For this review, take the finished solid that the model builds, in its own axes (mm). Coordinates: 2 decimals unless noted, no trailing zeros. Write each loop counter-clockwise with the first axis right and the second up, starting at its lowest first coordinate (ties: lowest second). Pieces come first, ordered by that corner, then holes. Notation, with made-up numbers: M 51,-26 L 97,-26 A13 cw 97,-16 Z; hole C -4,15 d2. An arc over 180 degrees is marked long. One line per question, with ' | ' between items.
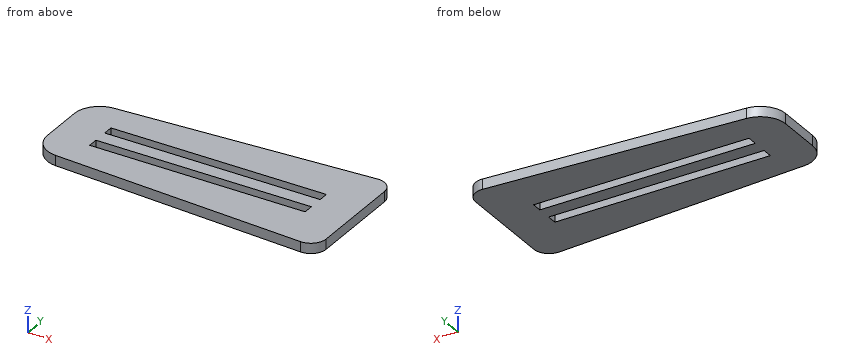
from build123d import *

# Parameters (mm, degrees)
F0_W     = 42.4481438452
F0_H     = 2
F1_DEPTH = 2
F2_R     = 3
F3_R     = 5


with BuildPart() as f1:
    # F0 (on Top) → F1 (new body)
    with BuildSketch(Plane.XY):
        Polygon((-65.7136544558, 44.0634722376), (-65.7136544558, 36.4734722376), (-65.7136544558, 35.0634722376), (-65.7136544558, 33.6534722376), (-65.7136544558, 26.0634722376), (-7.7136544558, 22.5634722376), (-7.7136544558, 47.5634722376), align=None)
        with Locations((-36.7136544558, 32.6534722376)):
            Rectangle(F0_W, F0_H, mode=Mode.SUBTRACT)
        with Locations((-36.7136544558, 37.4734722376)):
            Rectangle(F0_W, F0_H, mode=Mode.SUBTRACT)
    extrude(amount=F1_DEPTH)

    # F2
    f2_edges = [f1.edges().sort_by_distance(p)[0] for p in [
        (-7.713654, 47.563472, 1),
        (-7.713654, 22.563472, 1),
    ]]
    fillet(f2_edges, radius=F2_R)

    # F3
    f3_edges = [f1.edges().sort_by_distance(p)[0] for p in [
        (-65.713654, 26.063472, 1),
        (-65.713654, 44.063472, 1),
    ]]
    fillet(f3_edges, radius=F3_R)


solid = f1.part
1) We need section A-A on y = 37.5. State the section outline as (x, z) points, then the cut area to 3 significant figures.
Responses:
outline: M -65.71,0 L -57.94,0 L -57.94,2 L -65.71,2 Z; M -15.49,0 L -7.71,0 L -7.71,2 L -15.49,2 Z | area: 31.1 mm^2
2) We need section B-B on z = 1.3. State the section outline as (x, y) points.
Responses:
outline: M -65.71,30.77 A5 ccw -61.01,25.78 L -10.89,22.76 A3 ccw -7.71,25.75 L -7.71,44.38 A3 ccw -10.89,47.37 L -61.01,44.35 A5 ccw -65.71,39.36 Z; hole M -57.94,31.65 L -15.49,31.65 L -15.49,33.65 L -57.94,33.65 Z; hole M -57.94,36.47 L -15.49,36.47 L -15.49,38.47 L -57.94,38.47 Z
3) We need section C-C on x = -37. State the section outline as (y, z) points, then the cut area to 3 significant figures.
Responses:
outline: M 24.33,0 L 31.65,0 L 31.65,2 L 24.33,2 Z; M 33.65,0 L 36.47,0 L 36.47,2 L 33.65,2 Z; M 38.47,0 L 45.8,0 L 45.8,2 L 38.47,2 Z | area: 34.9 mm^2
4) To check wall thickness, follow line 1 along Y through (x, z) = (-37, 1.65); line 2 along Y through (x, z) = (-35.5, 0.55); line 3 along X through (y, z) = (27.5, 0.95). State the ranges of each line that lie inside material, in increasing order. Write a range as [from, to].
Responses:
line 1: [24.33, 31.65], [33.65, 36.47], [38.47, 45.8] | line 2: [24.24, 31.65], [33.65, 36.47], [38.47, 45.89] | line 3: [-64.5, -7.71]
5) Insertion check: pin 1 Ø0.6 at (x, z) = (-26.5, 1) entering from -Y; pin 2 Ø1.5 at (x, y) = (-23, 32) entering from -Z; pin 3 Ø1 at (y, z) = (44, 1) entering from -X; pin 4 Ø0.6 at (x, z) = (-39, 1) entering from +Y. Each pin has a flat end and moves straight along its axis. Give the tip position at first contact, or say it passes through.
Responses:
pin 1: y = 23.68 | pin 2: z = 0 | pin 3: x = -63.51 | pin 4: y = 45.69
6) We need section D-D on x = -57. State the section outline as (y, z) points.
Responses:
outline: M 25.54,0 L 31.65,0 L 31.65,2 L 25.54,2 Z; M 33.65,0 L 36.47,0 L 36.47,2 L 33.65,2 Z; M 38.47,0 L 44.59,0 L 44.59,2 L 38.47,2 Z
